Part model, mm, in its own coordinate system. Face numbers are marked on the shaded views. A direction names the side the tool comes from. Give positions to 0.01 mm unless a question says otherwise; leave off trailing zeros. Order: outer loops, then holes, each group sorted by start corner. A loop starts at its lowest first (then second) coordinate and runs counter-clockwise, first axis right, second up. Notation, with made-up numbers: M -22.75,62 L -14.75,62 A20 ccw -14.75,67 Z; hole C 38.25,-26 d5. An arc over 180 degrees is marked long. Return JSON: item names as keys, results as strings.
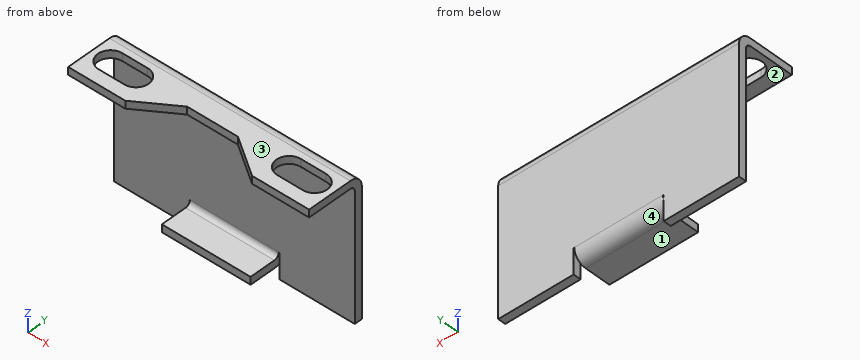
from build123d import *

# Parameters (mm, degrees)
BRIDA_BASE1_DEPTH                = 1.2
BRIDA_DE_ARISTA1_STRIP_W         = 6.2732
BRIDA_DE_ARISTA1_STRIP_H         = 1.2
BRIDA_DE_ARISTA1_STRIP_CUT_DEPTH = 38
BRIDA_DE_ARISTA1_DEPTH           = 38
BRIDA_DE_ARISTA2_STRIP_W         = 6.2732
BRIDA_DE_ARISTA2_STRIP_H         = 1.2
BRIDA_DE_ARISTA2_STRIP_CUT_DEPTH = 38
BRIDA_DE_ARISTA2_DEPTH           = 38
DESDOBLAR1_START                 = -19
DESDOBLAR1_DEPTH                 = 38
DESDOBLAR1_2_DEPTH               = 38
CROQUIS14_W                      = 12
CROQUIS14_H                      = 6.162926371
CORTAR_EXTRUIR1_DEPTH            = 1.2
DOBLAR1_START                    = -19
DOBLAR1_DEPTH                    = 38
DOBLAR1_2_DEPTH                  = 38
DOBLAR1_START_2                  = -7
DOBLAR1_3_DEPTH                  = 14
CROQUIS16_W                      = 11.9
CROQUIS16_H                      = 4
SALIENTE_EXTRUIR1_DEPTH          = 1.2


# Read off the part's stored shape, not the designer's step: Desdoblar1, Doblar1
# Sheet-metal steps are written as plain solids
with BuildPart() as part:
    # Croquis1 → Brida base1 (new body)
    with BuildSketch(Plane.XY):
        Polygon((-19, 19), (19, 19), (19, 10), (10, 10), (4, 14.085), (-4, 14.085), (-10, 10), (-19, 10), align=None)
        with BuildLine():
            Line((-16.085, 16.085), (-12.085, 16.085))
            ThreePointArc((-12.085, 16.085), (-10.085, 14.085), (-12.085, 12.085))
            Line((-12.085, 12.085), (-16.085, 12.085))
            ThreePointArc((-16.085, 12.085), (-18.085, 14.085), (-16.085, 16.085))
        make_face(mode=Mode.SUBTRACT)
        with BuildLine():
            Line((12.085, 16.085), (16.085, 16.085))
            ThreePointArc((16.085, 16.085), (18.085, 14.085), (16.085, 12.085))
            Line((16.085, 12.085), (12.085, 12.085))
            ThreePointArc((12.085, 12.085), (10.085, 14.085), (12.085, 16.085))
        make_face(mode=Mode.SUBTRACT)
    extrude(amount=-BRIDA_BASE1_DEPTH)

    # Brida de arista1 strip (across the edge) → Brida de arista1 strip cut (cut)
    with BuildSketch(Plane(origin=(-19, 19, -1.2), x_dir=(0, -1, 0), z_dir=(1, 0, 0))):
        with Locations((-1.2, -0.6)):
            Rectangle(BRIDA_DE_ARISTA1_STRIP_W, BRIDA_DE_ARISTA1_STRIP_H)
    extrude(amount=BRIDA_DE_ARISTA1_STRIP_CUT_DEPTH, mode=Mode.SUBTRACT)

    # Brida de arista1 section (across the edge) → Brida de arista1 (add)
    with BuildSketch(Plane(origin=(-19, 19, -1.2), x_dir=(0, -1, 0), z_dir=(1, 0, 0))):
        with BuildLine():
            Line((0, 0.7366), (0, 18.8))
            Line((0, 18.8), (1.2, 18.8))
            Line((1.2, 18.8), (1.2, 0.7366))
            ThreePointArc((1.2, 0.7366), (1.415745145, 0.215745145), (1.9366, 0))
            Line((1.9366, 0), (1.9366, -1.2))
            ThreePointArc((1.9366, -1.2), (0.567217008, -0.632782992), (0, 0.7366))
        make_face()
    extrude(amount=BRIDA_DE_ARISTA1_DEPTH)

    # Brida de arista2 strip (across the edge) → Brida de arista2 strip cut (cut)
    with BuildSketch(Plane(origin=(-19, 17.8, -20), x_dir=(0, 0, 1), z_dir=(1, 0, 0))):
        with Locations((-1.2, -0.6)):
            Rectangle(BRIDA_DE_ARISTA2_STRIP_W, BRIDA_DE_ARISTA2_STRIP_H)
    extrude(amount=BRIDA_DE_ARISTA2_STRIP_CUT_DEPTH, mode=Mode.SUBTRACT)

    # Brida de arista2 section (across the edge) → Brida de arista2 (add)
    with BuildSketch(Plane(origin=(-19, 17.8, -20), x_dir=(0, 0, 1), z_dir=(1, 0, 0))):
        with BuildLine():
            Line((0, 0.7366), (0, 4.8))
            Line((0, 4.8), (1.2, 4.8))
            Line((1.2, 4.8), (1.2, 0.7366))
            ThreePointArc((1.2, 0.7366), (1.415745145, 0.215745145), (1.9366, 0))
            Line((1.9366, 0), (1.9366, -1.2))
            ThreePointArc((1.9366, -1.2), (0.567217008, -0.632782992), (0, 0.7366))
        make_face()
    extrude(amount=BRIDA_DE_ARISTA2_DEPTH)

    # Desdoblar1 outline → Desdoblar1 (cut)
    with BuildSketch(Plane.YZ.offset(DESDOBLAR1_START)):
        with BuildLine():
            ThreePointArc((19, -1.9366), (18.963262642, -1.561178238), (18.854444388, -1.2))
            Line((18.854444388, -1.2), (17.0634, -1.2))
            ThreePointArc((17.0634, -1.2), (17.584254855, -1.415745145), (17.8, -1.9366))
            Line((17.8, -1.9366), (17.8, -18.0634))
            ThreePointArc((17.8, -18.0634), (17.584254855, -18.584254855), (17.0634, -18.8))
            Line((17.0634, -18.8), (13, -18.8))
            Line((13, -18.8), (13, -20))
            Line((13, -20), (17.0634, -20))
            ThreePointArc((17.0634, -20), (18.432782992, -19.432782992), (19, -18.0634))
            Line((19, -18.0634), (19, -1.9366))
        make_face()
    extrude(amount=DESDOBLAR1_DEPTH, mode=Mode.SUBTRACT)

    # Desdoblar1 2 outline → Desdoblar1 2 (add)
    with BuildSketch(Plane.YZ.offset(DESDOBLAR1_START)):
        with BuildLine():
            Line((41.452652741, 0), (17.0634, 0))
            ThreePointArc((17.0634, 0), (18.141342484, -0.327730969), (18.854444388, -1.2))
            Line((18.854444388, -1.2), (41.452652741, -1.2))
            Line((41.452652741, -1.2), (41.452652741, 0))
        make_face()
    extrude(amount=DESDOBLAR1_2_DEPTH)

    # Croquis14 → Cortar-Extruir1 (cut)
    with BuildSketch(Plane(origin=(0, 0, -1.2), x_dir=(-1, 0, 0), z_dir=(0, 0, -1))):
        with Locations((13, 38.371189556)):
            Rectangle(CROQUIS14_W, CROQUIS14_H)
        with Locations((-13, 38.371189556)):
            Rectangle(CROQUIS14_W, CROQUIS14_H)
    extrude(amount=-CORTAR_EXTRUIR1_DEPTH, mode=Mode.SUBTRACT)

    # Doblar1 outline → Doblar1 (cut)
    with BuildSketch(Plane.YZ.offset(DOBLAR1_START)):
        with BuildLine():
            ThreePointArc((17.0634, 0), (18.141342484, -0.327730969), (18.854444388, -1.2))
            Line((18.854444388, -1.2), (41.452652741, -1.2))
            Line((41.452652741, -1.2), (41.452652741, 0))
            Line((41.452652741, 0), (17.0634, 0))
        make_face()
    extrude(amount=DOBLAR1_DEPTH, mode=Mode.SUBTRACT)

    # Doblar1 2 outline → Doblar1 2 (add)
    with BuildSketch(Plane.YZ.offset(DOBLAR1_START)):
        with BuildLine():
            Line((19, -18.0634), (19, -1.9366))
            ThreePointArc((19, -1.9366), (18.963262642, -1.561178238), (18.854444388, -1.2))
            Line((18.854444388, -1.2), (17.0634, -1.2))
            ThreePointArc((17.0634, -1.2), (17.584254855, -1.415745145), (17.8, -1.9366))
            Line((17.8, -1.9366), (17.8, -18.0634))
            Line((17.8, -18.0634), (19, -18.0634))
        make_face()
    extrude(amount=DOBLAR1_2_DEPTH)

    # Doblar1 3 outline → Doblar1 3 (add)
    with BuildSketch(Plane.YZ.offset(DOBLAR1_START_2)):
        with BuildLine():
            ThreePointArc((17.0634, -20), (18.432782992, -19.432782992), (19, -18.0634))
            Line((19, -18.0634), (17.8, -18.0634))
            ThreePointArc((17.8, -18.0634), (17.584254855, -18.584254855), (17.0634, -18.8))
            Line((17.0634, -18.8), (13, -18.8))
            Line((13, -18.8), (13, -20))
            Line((13, -20), (17.0634, -20))
        make_face()
    extrude(amount=DOBLAR1_3_DEPTH)

    # Croquis16 → Saliente-Extruir1 (add)
    with BuildSketch(Plane(origin=(0, 19, 0), x_dir=(1, 0, 0), z_dir=(0, 1, 0))):
        with Locations((-13.05, 20.0634)):
            Rectangle(CROQUIS16_W, CROQUIS16_H)
        with Locations((13.05, 20.0634)):
            Rectangle(CROQUIS16_W, CROQUIS16_H)
    extrude(amount=-SALIENTE_EXTRUIR1_DEPTH)


solid = part.part
Q1. Band-saw the part on D-D (x = -11.5). Give the cut face in (y, z), then the cut area to 3 significant figures.
Established:
{"outline": "M 10,-1.2 L 12.17,-1.2 L 12.17,0 L 10,0 Z; M 16,-1.2 L 17.06,-1.2 A0.74 cw 17.8,-1.94 L 17.8,-22.06 L 19,-22.06 L 19,-1.94 A1.94 ccw 17.06,0 L 16,0 Z", "area": "30.6 mm²"}
Q2. Pin check, flat tips, straight feed: pin 1 (1 mm diameter, centred on x = -13.5, z = -1, fed in from +Y); pin 2 (5 mm diameter, centred on x = -11.5, z = -4, fed in from -Y); pin 3 (2 mm diameter, centred on y = 14.5, z = -19.5, fed in from -X). Stop position of each tip, or through.
Established:
{"pin 1": "stops at y = 18.95", "pin 2": "stops at y = 17.66", "pin 3": "stops at x = -7"}
Q3. Probe line 1 along Z through (x, y) = (1, 16); line 2 along Y through (x, z) = (3.5, -11.5); line 3 along Z through (x, y) = (-9.5, 14). List the from-to ranges inside material, lowest first.
Established:
{"line 1": "z = -20 to -18.8, -1.2 to 0", "line 2": "y = 17.8 to 19", "line 3": "z = -1.2 to 0"}
Q4. Two-plate mould, pull along X, no slides. Class the marked faces 3 and 4: +X half, -X half, draft (parallel to the pull), parting line (faces both ways), or undercut.
Established:
{"face 3": "draft", "face 4": "undercut"}
Q5. Band-saw the part on C-C (x = -1.5). Give the cut face in (y, z) (3 decimals), then the cut area to 3 significant figures.
Established:
{"outline": "M 13,-20 L 17.063,-20 A1.937 ccw 19,-18.063 L 19,-1.937 A1.937 ccw 17.063,0 L 14.085,0 L 14.085,-1.2 L 17.063,-1.2 A0.737 cw 17.8,-1.937 L 17.8,-18.063 A0.737 cw 17.063,-18.8 L 13,-18.8 Z", "area": "32.8 mm²"}
Q6. 3-axis set-ups, long thin cutter, end or side, ignore diameter. For the marked faces 1 and 2: which of +Z, -Z, +X, -X, +Y, -Y reach the whole face in a straight line?
Established:
{"face 1": "-Z, +X, -X, +Y, -Y", "face 2": "+X, -X, -Y"}
Q7. Band-saw the part on B-B (y = 16.5). Give the cut face in (x, z), then the cut area to 3 significant figures.
Established:
{"outline": "M -19,-1.2 L 19,-1.2 L 19,0 L -19,0 Z; M -7,-20 L 7,-20 L 7,-18.8 L -7,-18.8 Z", "area": "62.4 mm²"}
Q8. Band-saw the part on A-A (x = 14.5). Give the cut face in (y, z) (3 decimals).
Established:
{"outline": "M 10,-1.2 L 12.085,-1.2 L 12.085,0 L 10,0 Z; M 16.085,-1.2 L 17.063,-1.2 A0.737 cw 17.8,-1.937 L 17.8,-22.063 L 19,-22.063 L 19,-1.937 A1.937 ccw 17.063,0 L 16.085,0 Z"}
